Check sheet for the modelled part. Datum: model origin and axes. Units: mm. A direction names the side the tool comes from. Round coordinates to 2 decimals unless told otherwise and drop trailing zeros. Order: outer loops, then holes, each group sorted by start corner. A loop starts at its lowest first (then second) coordinate and runs counter-clockwise, first axis right, second up. Notation, with made-up numbers: (2, 46) -> (50, 46) arc R23 ccw to (50, 75) -> close; hole circle Ø7 at (29, -12). An arc over 180 degrees is marked (long way). Use CSV: the item, a comma, the result in double quotes.
```python
from build123d import *

# Parameters (mm, degrees)
F0_R     = 10.9855
F1_DEPTH = 37.592
F2_W     = 12.7
F2_H     = 3.175
F3_DEPTH = 10.922
F4_R     = 0.5518892204


with BuildPart() as f1:
    # F0 (on Right) → F1 (new body, symmetric)
    with BuildSketch(Plane.YZ):
        Circle(F0_R)
    extrude(amount=F1_DEPTH, both=True)

    # F2 (on face) → F3 (cut)
    with BuildSketch(Plane.YZ.offset(37.592)):
        with Locations((0, 1.778)):
            Rectangle(F2_W, F2_H)
    extrude(amount=-F3_DEPTH, mode=Mode.SUBTRACT)

    # F4
    f4_edges = [f1.edges().sort_by_distance(p)[0] for p in [
        (37.592, -10.9855, 0),
        (-37.592, -10.9855, 0),
    ]]
    fillet(f4_edges, radius=F4_R)


solid = f1.part
```
Q1. Sectioned sample at B-B, the plane x = -0.5. Enter the section's corners in (y, z), then the cut area to 3 significant figures.
Result sheet:
outline,"circle Ø21.97 at (0, 0)"
area,"379 mm^2"
Q2. Mould release check, pull along Y, two halves, no side actions. Record for faces 1 (the face through (32, 0, 0.191)), 2 (the face through (-37.592, 0, 0)), 3 (the face through (26.67, 0, 2)), 4 (the face through (0.52, 10.48, 3.3)): pulls with the +Y half, pulls with the -Y half, needs draft (parallel to the pull), parting line crosses it, or undercut.
Result sheet:
face 1,"undercut"
face 2,"needs draft"
face 3,"undercut"
face 4,"parting line crosses it"
Q3. Access from +Z, -Z, +X, -X, +Y, -Y to the whole of each face (thin tool, end or side, straight path). Record for faces 5 (the face through (32, 6.35, 2)), 6 (the face through (37.592, 0, 0)).
Result sheet:
face 5,"+X"
face 6,"+Z, -Z, +X, +Y, -Y"
Q4. Scan lines: L1, parallel to Z at x = 25.5, y = 0; L2, parallel to X at y = -1.25, z = 1.5; L3, parallel to Y at x = -18, z = 0.5. Record each from-to range of solid material in increasing order.
Result sheet:
L1,"z = -10.99 to 10.99"
L2,"x = -37.59 to 26.67"
L3,"y = -10.97 to 10.97"
Q5. Go/stop test with flat-tipped pins: pin 1 (2 mm diameter, centred on x = -2.5, y = -6, fed in from -Z); pin 2 (8 mm diameter, centred on x = -21.5, z = 7.5, fed in from +Y); pin 3 (6 mm diameter, centred on x = 18, z = 7, fed in from -Y). Record where each tip stops, or that it passes through.
Result sheet:
pin 1,"stops at z = -9.78"
pin 2,"stops at y = 10.41"
pin 3,"stops at y = -10.23"
Q6. Sectioned sample at A-A, the plane y = 0. Enter the section's corners in (x, z), then the cut area to 3 significant figures.
Result sheet:
outline,"(-37.59, -10.43) arc R0.55 ccw to (-37.04, -10.99) -> (37.04, -10.99) arc R0.55 ccw to (37.59, -10.43) -> (37.59, 0.19) -> (26.67, 0.19) -> (26.67, 3.37) -> (37.59, 3.37) -> (37.59, 10.43) arc R0.55 ccw to (37.04, 10.99) -> (-37.04, 10.99) arc R0.55 ccw to (-37.59, 10.43) -> close"
area,"1,620 mm^2"
